Here's how the part is built. I have some questions about the finished solid (model axes, mm). Give positions to 0.01 mm unless a question says otherwise; leave off trailing zeros. Write each loop counter-clockwise with the first axis right and the second up, starting at its lowest first coordinate (ties: lowest second). Pieces come first, ordered by that corner, then holes. Notation, with made-up numbers: (30, 2.5) - (77, 2.5) arc R18 cw to (77, 25.5) - close; hole circle Ø8 at (73.5, 84.5). An arc over 180 degrees is marked (long way). Use one line per item in the form item = value. Start each with the question number.
Autodesk Inventor part; units mm, degrees
ref_plane "YZ Plane" through (0, 0, 0) normal (1, 0, 0) x (0, 1, 0)
ref_plane "XZ Plane" through (0, 0, 0) normal (0, 1, 0) x (-1, 0, 0)
ref_plane "XY Plane" through (0, 0, 0) normal (0, 0, 1) x (1, 0, 0)
sketch "Sketch1" plane through (0, 0, 0) normal (0, 1, 0) x (-1, 0, 0)
  circle A0 centre (0, 0) radius 5.7
  arc A1 (0, 9) -> (0, -9) centre (0, 0) ccw construction
  line L0 (0, 9) -> (12.65, 9) construction
  line L1 (12.65, 9) -> (12.65, -9) construction
  line L2 (0, 0) -> (0, -9) construction
  line L3 (3.0786, -10) -> (30, -10)
  line L4 (35, -5) -> (35, 5)
  line L5 (30, 10) -> (3.0786, 10)
  arc A2 (35, 5) -> (30, 10) centre (30, 5) ccw
  arc A3 (30, -10) -> (35, -5) centre (30, -5) ccw
  line L6 (2.8334, -9.9925) -> (-0.6007, -9.7816)
  line L7 (2.8334, 9.9925) -> (-0.6007, 9.7816)
  arc A4 (2.8334, -9.9925) -> (3.0786, -10) centre (3.0786, -6) ccw
  arc A5 (3.0786, 10) -> (2.8334, 9.9925) centre (3.0786, 6) ccw
  line L8 (0, 0) -> (36.2824, 0)
  line L9 (-9, 3.8781) -> (-9, -3.8781)
  arc A6 (-0.6007, 9.7816) -> (-9, 3.8781) centre (0, 0) ccw
  arc A7 (-9, -3.8781) -> (-0.6007, -9.7816) centre (0, 0) ccw
  point P0 (35, -10)
  point P1 (35, 10)
  point P2 (2, -10)
  point P3 (2.9559, 10)
  dimension "d0" = 11.4
  dimension "d1" = 9
  dimension "d2" = 12.65
  dimension "d6" = 5
  dimension "d10" = 20
  dimension "d12" = 4
  dimension "d13" = 20
  dimension "d14" = 20
extrude "Extrusion1" add sketch "Sketch1" along normal blind 0.5
properties part number "Laser-Pivot-Ringpull"
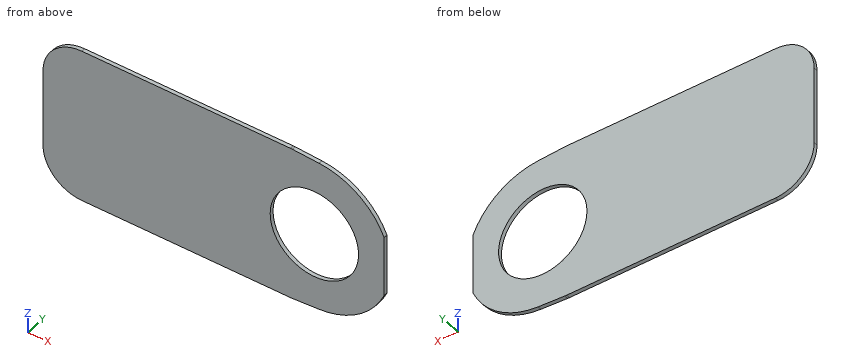
1. I want a section at C-C, the plane x = 0. List the corners of the cut face in (y, z) for me, then the cut area to 3 significant figures.
2. I want a section at B-B, the plane z = 0. List the corners of the cut face in (x, y) for me, then the cut area to 3 significant figures.
3. I want a section at A-A, the plane y = 0.2. List the corners of the cut face in (x, z) for me, then the cut area to 3 significant figures.
4. I want a section at D-D, the plane z = 6.5. List the corners of the cut face in (x, y) for me, then the cut area to 3 significant figures.
5. Please list where these lines run through material, in increasing order: line 1 (Z direction, x = 0, y = 0.2); line 2 (Z direction, x = 2, y = 0.1); line 3 (X direction, y = 0.45, z = 4.25).
Result sheet:
q1.outline = (0, -9.82) - (0.5, -9.82) - (0.5, -5.7) - (0, -5.7) - close; (0, 5.7) - (0.5, 5.7) - (0.5, 9.82) - (0, 9.82) - close
q1.area = 4.12 mm2
q2.outline = (-35, 0) - (-5.7, 0) - (-5.7, 0.5) - (-35, 0.5) - close; (5.7, 0) - (9, 0) - (9, 0.5) - (5.7, 0.5) - close
q2.area = 16.3 mm2
q3.outline = (-35, -5) arc R5 ccw to (-30, -10) - (-3.08, -10) arc R3.98 ccw to (-2.83, -9.99) - (0.6, -9.78) arc R9.8 ccw to (9, -3.88) - (9, 3.88) arc R9.8 ccw to (0.6, 9.78) - (-2.83, 9.99) arc R4.02 ccw to (-3.08, 10) - (-30, 10) arc R5 ccw to (-35, 5) - close; hole circle Ø11.4 at (0, 0)
q3.area = 733 mm2
q4.outline = (-34.77, 0) - (7.33, 0) - (7.33, 0.5) - (-34.77, 0.5) - close
q4.area = 21.1 mm2
q5.line_1 = -9.82 to -5.7, 5.7 to 9.82
q5.line_2 = -9.59 to -5.34, 5.34 to 9.59
q5.line_3 = -35 to -3.8, 3.8 to 8.83
